```python
from build123d import *

# Parameters (mm, degrees)
SKETCH1_R           = 2
SKETCH1_R_2         = 6.35
SKETCH1_R_3         = 1.905
SKETCH1_R_4         = 2.575
SKETCH1_W           = 21.082
SKETCH1_H           = 40.64
BOSS_EXTRUDE1_DEPTH = 3.175


with BuildPart() as part:
    # Sketch1 → Boss-Extrude1 (new, symmetric)
    with BuildSketch(Plane.XY):
        with BuildLine():
            Line((-16.129, -83.74), (16.129, -83.74))
            ThreePointArc((16.129, -83.74), (19.721102448, -82.252102448), (21.209, -78.66))
            Line((21.209, -78.66), (21.209, 18.542))
            ThreePointArc((21.209, 18.542), (22.696897552, 22.134102448), (26.289, 23.622))
            Line((26.289, 23.622), (30.099, 23.622))
            ThreePointArc((30.099, 23.622), (33.691102448, 25.109897552), (35.179, 28.702))
            Line((35.179, 28.702), (35.179, 73.66))
            ThreePointArc((35.179, 73.66), (33.691102448, 77.252102448), (30.099, 78.74))
            Line((30.099, 78.74), (-30.099, 78.74))
            ThreePointArc((-30.099, 78.74), (-33.691102448, 77.252102448), (-35.179, 73.66))
            Line((-35.179, 73.66), (-35.179, 28.702))
            ThreePointArc((-35.179, 28.702), (-33.691102448, 25.109897552), (-30.099, 23.622))
            Line((-30.099, 23.622), (-26.289, 23.622))
            ThreePointArc((-26.289, 23.622), (-22.696897552, 22.134102448), (-21.209, 18.542))
            Line((-21.209, 18.542), (-21.209, -78.66))
            ThreePointArc((-21.209, -78.66), (-19.721102448, -82.252102448), (-16.129, -83.74))
        make_face()
        with Locations((8.4836, 11.938)):
            Circle(SKETCH1_R, mode=Mode.SUBTRACT)
        with Locations((-8.5344, 11.938)):
            Circle(SKETCH1_R, mode=Mode.SUBTRACT)
        with Locations((-8.5344, -11.938)):
            Circle(SKETCH1_R, mode=Mode.SUBTRACT)
        with Locations((8.4836, -11.938)):
            Circle(SKETCH1_R, mode=Mode.SUBTRACT)
        with Locations((0, 51.181)):
            Circle(SKETCH1_R_2, mode=Mode.SUBTRACT)
        with Locations((15.494, 66.675)):
            Circle(SKETCH1_R_3, mode=Mode.SUBTRACT)
        with Locations((-15.494, 66.675)):
            Circle(SKETCH1_R_3, mode=Mode.SUBTRACT)
        with Locations((-15.494, 35.687)):
            Circle(SKETCH1_R_3, mode=Mode.SUBTRACT)
        with Locations((15.494, 35.687)):
            Circle(SKETCH1_R_3, mode=Mode.SUBTRACT)
        with Locations((-5.1689, -26.32)):
            Circle(SKETCH1_R, mode=Mode.SUBTRACT)
        with Locations((5.2451, -26.32)):
            Circle(SKETCH1_R, mode=Mode.SUBTRACT)
        with Locations((5.2451, -76.104)):
            Circle(SKETCH1_R, mode=Mode.SUBTRACT)
        with Locations((-5.1689, -76.104)):
            Circle(SKETCH1_R, mode=Mode.SUBTRACT)
        with Locations((-26.67, 51.181)):
            Circle(SKETCH1_R_4, mode=Mode.SUBTRACT)
        with Locations(Location((26.67, 51.181, 0), (0, 0, 180))):
            Circle(SKETCH1_R_4, mode=Mode.SUBTRACT)
        with BuildLine():
            Line((7.723020264, 60.700071488), (10.237491978, 63.214543202))
            ThreePointArc((10.237491978, 63.214543202), (12.033543202, 63.214543202), (12.033543202, 61.418491978))
            Line((12.033543202, 61.418491978), (9.519071488, 58.904020264))
            ThreePointArc((9.519071488, 58.904020264), (7.723020264, 58.904020264), (7.723020264, 60.700071488))
        make_face(mode=Mode.SUBTRACT)
        with BuildLine():
            Line((-9.519071488, 58.904020264), (-12.033543202, 61.418491978))
            ThreePointArc((-12.033543202, 61.418491978), (-12.033543202, 63.214543202), (-10.237491978, 63.214543202))
            Line((-10.237491978, 63.214543202), (-7.723020264, 60.700071488))
            ThreePointArc((-7.723020264, 60.700071488), (-7.723020264, 58.904020264), (-9.519071488, 58.904020264))
        make_face(mode=Mode.SUBTRACT)
        with Locations((0, -51.212)):
            Rectangle(SKETCH1_W, SKETCH1_H, mode=Mode.SUBTRACT)
        with BuildLine():
            Line((-7.723020264, 41.661928512), (-10.237491978, 39.147456798))
            ThreePointArc((-10.237491978, 39.147456798), (-12.033543202, 39.147456798), (-12.033543202, 40.943508022))
            Line((-12.033543202, 40.943508022), (-9.519071488, 43.457979736))
            ThreePointArc((-9.519071488, 43.457979736), (-7.723020264, 43.457979736), (-7.723020264, 41.661928512))
        make_face(mode=Mode.SUBTRACT)
        with BuildLine():
            Line((9.519071488, 43.457979736), (12.033543202, 40.943508022))
            ThreePointArc((12.033543202, 40.943508022), (12.033543202, 39.147456798), (10.237491978, 39.147456798))
            Line((10.237491978, 39.147456798), (7.723020264, 41.661928512))
            ThreePointArc((7.723020264, 41.661928512), (7.723020264, 43.457979736), (9.519071488, 43.457979736))
        make_face(mode=Mode.SUBTRACT)
    extrude(amount=BOSS_EXTRUDE1_DEPTH, both=True)


solid = part.part
```
Model file for the job. Use its own axes, mm. A direction names the side the tool comes from. Coordinates: 2 decimals unless noted, no trailing zeros. Write each loop counter-clockwise with the first axis right and the second up, starting at its lowest first coordinate (ties: lowest second). Pieces come first, ordered by that corner, then holes. Notation, with made-up numbers: (49, -18.75) - (96, -18.75) arc R27 ccw to (96, 0.25) - close; hole circle Ø9 at (56.25, 4). An arc over 180 degrees is marked (long way). Use a Markdown table: item, result. Add a question column.
Item 1: Band-saw the part on D-D, the plane z = -1. Give the number of separate pieces and of enclosed holes in the cut face, and give its area (3 significant figures).
Item 2: Band-saw the part on A-A, the plane y = -44. Write the cut outline in (x, z) (3 decimals).
Item 3: Drop flat-ended pins along their axis: pin 1 (1.1 mm diameter, centred on x = -29, z = -0.5, fed in from -Y); pin 2 (2 mm diameter, centred on y = -51.5, z = -1.5, fed in from -X); pin 3 (1.9 mm diameter, centred on y = -58.5, z = -1.5, fed in from +X). Give the stop position or say it passes through.
Item 4: Band-saw the part on C-C, the plane y = -26.32. Write the cut outline in (x, z) (3 decimals).
Item 5: 3-axis set-ups, long thin cutter, end or side, ignore diameter. For faces 1 (the face through (-6.627, -11.337, -0.044)), 2 (the face through (-28, 23.622, 0)), 3 (the face through (21.209, -31, 0)): which of +Z, -Z, +X, -X, +Y, -Y reach the whole face in a straight line?
Item 6: Two-plate mould, pull along Y, no slides. Class faces 4 (the face through (33.73, 77.21, 0.04)), 5 (the face through (33.65, 25.07, 0.04)), 6 (the face through (10.541, -51, 0)): pulls with the +Y half, pulls with the -Y half, needs draft (parallel to the pull), parting line crosses it, or undercut.
Item 7: Drill centre lines: line 1 along Y through (x, z) = (0, 1.75); line 2 along Y through (x, z) = (26.5, 0); line 3 along X through (y, z) = (12.5, 2). Where is each one in solid material? Low to high.
Item 8: Band-saw the part on B-B, the plane x = 0. Write the cut outline in (y, z) (3 decimals), and give its area (3 significant figures).
A:
| question | item | result |
|---|---|---|
| 1 | separate pieces | 1 |
| 1 | enclosed holes | 20 |
| 1 | area | 7,180 mm² |
| 2 | outline | (-21.209, -3.175) - (-10.541, -3.175) - (-10.541, 3.175) - (-21.209, 3.175) - close; (10.541, -3.175) - (21.209, -3.175) - (21.209, 3.175) - (10.541, 3.175) - close |
| 3 | pin 1 | stops at y = 23.62 |
| 3 | pin 2 | stops at x = -21.21 |
| 3 | pin 3 | stops at x = 21.21 |
| 4 | outline | (-21.209, -3.175) - (-7.169, -3.175) - (-7.169, 3.175) - (-21.209, 3.175) - close; (-3.169, -3.175) - (3.245, -3.175) - (3.245, 3.175) - (-3.169, 3.175) - close; (7.245, -3.175) - (21.209, -3.175) - (21.209, 3.175) - (7.245, 3.175) - close |
| 5 | face 1 | +Z, -Z |
| 5 | face 2 | +Z, -Z, -X, -Y |
| 5 | face 3 | +Z, -Z, +X, -Y |
| 6 | face 4 | pulls with the +Y half |
| 6 | face 5 | pulls with the -Y half |
| 6 | face 6 | undercut |
| 7 | line 1 | y = -83.74 to -71.53, -30.89 to 44.83, 57.53 to 78.74 |
| 7 | line 2 | y = 23.62 to 48.61, 53.75 to 78.74 |
| 7 | line 3 | x = -21.21 to -10.45, -6.61 to 6.56, 10.4 to 21.21 |
| 8 | outline | (-83.74, -3.175) - (-71.532, -3.175) - (-71.532, 3.175) - (-83.74, 3.175) - close; (-30.892, -3.175) - (44.831, -3.175) - (44.831, 3.175) - (-30.892, 3.175) - close; (57.531, -3.175) - (78.74, -3.175) - (78.74, 3.175) - (57.531, 3.175) - close |
| 8 | area | 693 mm² |
